For this review, use the dimensioned drawing (mm, ordinates from the lowest corner) and the shaded views. A direction names the side the tool comes from. Round coordinates to 2 decimals unless told otherwise and drop trailing zeros. Loops run counter-clockwise (first coordinate to the right, second up) from the corner with the lowest first, then second, coordinate; pieces in that order, holes last. Notation, with made-up numbers: M 88.5,-8 L 129.5,-8 A25 cw 129.5,13 Z; hole C 87,40.5 d5. An arc over 180 degrees is marked long. One line per item, written item: value. Start each with the question number.
Item 1: Clearance check with flat-ended pins moving along their axes: pin 1 (8 mm diameter, centred on y = 88, z = 24.5, fed in from -X); pin 2 (7.5 mm diameter, centred on x = 9.5, y = 71.5, fed in from +Z). State where each tip first meets the part, or that it passes through.
Item 2: We need section D-D (y = 11). Write out the cut boundary in (x, z).
Item 3: For line 1 along Y through (x, z) = (49.5, 33); line 2 along X through (y, z) = (4.5, 41.5); line 3 along Z through (x, y) = (22, 47.5), list the stretches that pass through material, from the lowest coordinate up.
Item 4: Mouldability with a two-part tool opening along Y and no side actions: class the marked faces 5, 6 and 7 as released by +Y, released by -Y, zero draft, split by the parting line, or undercut.
Item 5: We need section C-C (z = 13). Write out the cut boundary in (x, y), then the cut area to 3 significant figures.
Item 6: We need section A-A (y = 50). Write out the cut boundary in (x, z).
Item 7: For the marked faces 1, 2, 3 and 4, list the 3-axis set-ups (+Z, -Z, +X, -X, +Y, -Y) from which the entire face can be reached by the end or side of a thin tool; tool diameter is ignored.
Item 8: We need section B-B (x = 50). Write out the cut boundary in (y, z).
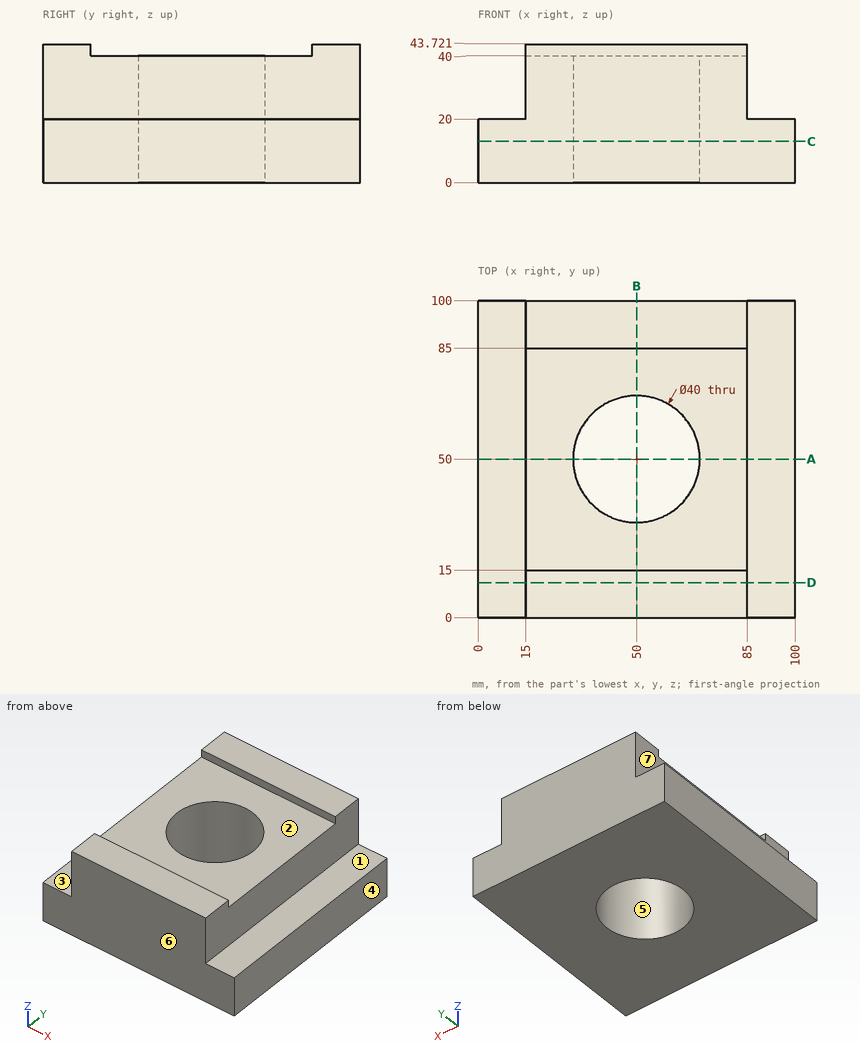
A:
1. pin 1: x = 15
1. pin 2: z = 20
2. outline: M 0,0 L 100,0 L 100,20 L 85,20 L 85,43.72 L 15,43.72 L 15,20 L 0,20 Z
3. line 1: 0 to 30.01, 69.99 to 100
3. line 2: 15 to 85
3. line 3: 0 to 40
4. face 5: undercut
4. face 6: released by -Y
4. face 7: zero draft
5. outline: M 0,0 L 100,0 L 100,100 L 0,100 Z; hole C 50,50 d40
5. area: 8,740 mm2
6. outline: M 0,0 L 30,0 L 30,40 L 15,40 L 15,20 L 0,20 Z; M 70,0 L 100,0 L 100,20 L 85,20 L 85,40 L 70,40 Z
7. face 1: +Z, +X, +Y, -Y
7. face 2: +Z, +X, -X
7. face 3: +Z, -X, +Y, -Y
7. face 4: +Z, -Z, +X, +Y, -Y
8. outline: M 0,0 L 30,0 L 30,40 L 15,40 L 15,43.72 L 0,43.72 Z; M 70,0 L 100,0 L 100,43.72 L 85,43.72 L 85,40 L 70,40 Z
